```python
from build123d import *

# Parameters (mm, degrees)
BOSS_EXTRU_1_DEPTH = 6


with BuildPart() as part:
    # Esquisse1 → Boss.-Extru.1 (new body)
    with BuildSketch(Plane.XY):
        with BuildLine():
            Line((-373.69467463, 106.042558597), (-365.69467463, 76.042558597))
            Line((-365.69467463, 76.042558597), (-365.69467463, -43.957441403))
            Line((-365.69467463, -43.957441403), (-373.69467463, -73.957441403))
            ThreePointArc((-373.69467463, -73.957441403), (-360.192601556, -108.141248671), (-326.969404712, -123.859322601))
            Line((-326.969404712, -123.859322601), (-296.875879039, -115.85986931))
            Line((-296.875879039, -115.85986931), (-76.875879039, -115.85986931))
            Line((-76.875879039, -115.85986931), (-46.969404712, -123.859322601))
            ThreePointArc((-46.969404712, -123.859322601), (-11.649350298, -109.24901926), (3.029605382, -73.957441403))
            Line((3.029605382, -73.957441403), (-4.970394618, -43.957441403))
            Line((-4.970394618, -43.957441403), (-4.970394618, 76.042558597))
            Line((-4.970394618, 76.042558597), (3.029605382, 106.042558597))
            ThreePointArc((3.029605382, 106.042558597), (-10.442134726, 140.284021287), (-43.697023707, 156.03451041))
            Line((-43.697023707, 156.03451041), (-73.79054938, 148.035057119))
            Line((-73.79054938, 148.035057119), (-293.79054938, 148.035057119))
            Line((-293.79054938, 148.035057119), (-323.697023707, 156.03451041))
            ThreePointArc((-323.697023707, 156.03451041), (-359.04799913, 141.391864616), (-373.69467463, 106.042558597))
        make_face()
    extrude(amount=BOSS_EXTRU_1_DEPTH)


solid = part.part
```
Geometry: final body of the model. Coordinates: model frame, mm. A direction names the side the tool comes from. Coordinates: 2 decimals unless noted, no trailing zeros. Order: outer loops, then holes, each group sorted by start corner. A loop starts at its lowest first (then second) coordinate and runs counter-clockwise, first axis right, second up. Notation, with made-up numbers: (25, 4.25) - (56, 4.25) arc R15 ccw to (56, 8.25) - close; hole circle Ø4 at (68, 16.5). An arc over 180 degrees is marked (long way). Write each question's results on one line, items separated by ' | '.
(1) First-contact query: pin 1 Ø1.8 at (x, z) = (-180.5, 2.5) entering from -Y; pin 2 Ø1.5 at (y, z) = (11, 3.5) entering from +X; pin 3 Ø1.8 at (y, z) = (-3, 3) entering from -X. Flat tips, straight axial feed; report the tip coordinate or a pass-through.
Values found:
pin 1: stops at y = -115.86 | pin 2: stops at x = -4.97 | pin 3: stops at x = -365.69
(2) Section query B-B, the plane y = -32.5. Return the cut outline in (x, z), plus the area to 3 significant figures.
Values found:
outline: (-365.69, 0) - (-4.97, 0) - (-4.97, 6) - (-365.69, 6) - close | area: 2,160 mm²
(3) Section query C-C, the plane x = -241.5. Return the cut outline in (y, z).
Values found:
outline: (-115.86, 0) - (148.04, 0) - (148.04, 6) - (-115.86, 6) - close
(4) Section query A-A, the plane z = 2.9. Return the cut outline in (x, y), plus the area to 3 significant figures.
Values found:
outline: (-373.69, -73.96) arc R50 ccw to (-326.97, -123.86) - (-296.88, -115.86) - (-76.88, -115.86) - (-46.97, -123.86) arc R50 ccw to (3.03, -73.96) - (-4.97, -43.96) - (-4.97, 76.04) - (3.03, 106.04) arc R50 ccw to (-43.7, 156.03) - (-73.79, 148.04) - (-293.79, 148.04) - (-323.7, 156.03) arc R50 ccw to (-373.69, 106.04) - (-365.69, 76.04) - (-365.69, -43.96) - close | area: 96,900 mm²
(5) Mould query, pull axis X, two halves, no side actions, for faces 1 (the face through (-12.04, -109.635, 2.958)), 2 (the face through (-188, 18, 0)), 3 (the face through (-62.132, -119.804, 2.958)), 4 (the face through (-358.657, 141.778, 2.958)). Classes: +X half, -X half, draft (parallel to the pull), parting line (faces both ways), or undercut.
Values found:
face 1: +X half | face 2: draft | face 3: undercut | face 4: -X half
(6) Line query: line 1 (X direction, y = -41.5, z = 2.45); line 2 (Y direction, x = -268, z = 2.9); line 3 (Y direction, x = -323, z = 2.8). Output: solid intervals per line, ascending. Write a range as [from, to].
Values found:
line 1: x = [-365.69, -4.97] | line 2: y = [-115.86, 148.04] | line 3: y = [-122.8, 155.85]
(7) Set-up query: faces 5 (the face through (-308.534, 151.979, 2.958)), 6 (the face through (-1.026, 90.833, 2.958)), 7 (the face through (-312.133, -119.916, 2.958)), 8 (the face through (-369.75, 91.25, 2.96)). Return all of +Z, -Z, +X, -X, +Y, -Y with unobstructed straight access to the full face (end or side cutting, diameter ignored); none if empty.
Values found:
face 5: +Z, -Z, +Y | face 6: +Z, -Z, +X | face 7: +Z, -Z, -Y | face 8: +Z, -Z, -X
